Check sheet for the modelled part. Datum: model origin and axes. Units: mm. A direction names the side the tool comes from. Round coordinates to 2 decimals unless told otherwise and drop trailing zeros. Order: outer loops, then holes, each group sorted by start corner. A loop starts at its lowest first (then second) coordinate and runs counter-clockwise, first axis right, second up.
(1) Sectioned sample at C-C, the plane y = 215.5. Enter the section's corners in (x, z).
(2) Thickness scan on probe 1 along X at (y, z) = (1386.5, 16); probe 2 along Z at (x, y) = (-38, 834). Record the ranges inside material, lowest first.
(3) Mould release check, pull along Z, two halves, no side actions. Record for faces 1 (the flat face through (-17.742, 806, 3)), 2 (the flat face through (-37, 806, -15.292)), 3 (the flat face through (-37, 806, 23.208)): released by +Z, released by -Z, zero draft, split by the parting line, or undercut.
(4) Sectioned sample at A-A, the plane x = -49. Enter the section's corners in (y, z).
(5) Sectioned sample at B-B, the plane z = 15. Enter the section's corners in (x, y).
(6) Tool access check on faces 4 (the flat face through (-19.242, 806, 3)), 5 (the flat face through (-57.742, 806, 3)). Record the directions out of +Z, -Z, +X, -X, +Y, -Y that give a thin tool (end or side, any length) a straight path to the whole face; none if there is none.
Autodesk Inventor part; units mm, degrees
ref_plane "YZ Plane" through (0, 0, 0) normal (1, 0, 0) x (0, 1, 0)
ref_plane "XZ Plane" through (0, 0, 0) normal (0, 1, 0) x (-1, 0, 0)
ref_plane "XY Plane" through (0, 0, 0) normal (0, 0, 1) x (1, 0, 0)
sketch "Sketch1" plane through (0, 0, 0) normal (0, 1, 0) x (-1, 0, 0)
  line L0 (18.2419, 23.2079) -> (57.2419, 23.2079)
  line L1 (57.7419, 22.7079) -> (57.7419, -16.2921)
  line L2 (57.2419, -16.7921) -> (18.2419, -16.7921)
  line L3 (17.7419, -16.2921) -> (17.7419, 22.7079)
  line L4 (56.2419, 21.7079) -> (19.2419, 21.7079)
  line L5 (19.2419, 21.7079) -> (19.2419, -15.2921)
  line L6 (19.2419, -15.2921) -> (56.2419, -15.2921)
  line L7 (56.2419, -15.2921) -> (56.2419, 21.7079)
  arc A0 (18.2419, 23.2079) -> (17.7419, 22.7079) centre (18.2419, 22.7079) ccw
  arc A1 (57.7419, 22.7079) -> (57.2419, 23.2079) centre (57.2419, 22.7079) ccw
  arc A2 (57.2419, -16.7921) -> (57.7419, -16.2921) centre (57.2419, -16.2921) ccw
  arc A3 (17.7419, -16.2921) -> (18.2419, -16.7921) centre (18.2419, -16.2921) ccw
  point P0 (0, 0)
  point P1 (17.7419, 23.2079)
  point P2 (57.7419, 23.2079)
  point P3 (57.7419, -16.7921)
  dimension "d0" = 40
  dimension "d1" = 40
  dimension "d2" = 1.5
  dimension "d3" = 0.5
extrude "Extrusion1" add sketch "Sketch1" along normal blind 1635
properties part number "Metalon_Base_2"
Derived:
1. outline: (-57.74, -16.29) arc R0.5 ccw to (-57.24, -16.79) - (-18.24, -16.79) arc R0.5 ccw to (-17.74, -16.29) - (-17.74, 22.71) arc R0.5 ccw to (-18.24, 23.21) - (-57.24, 23.21) arc R0.5 ccw to (-57.74, 22.71) - close; hole (-56.24, -15.29) - (-19.24, -15.29) - (-19.24, 21.71) - (-56.24, 21.71) - close
2. probe 1: x = -57.74 to -56.24, -19.24 to -17.74
2. probe 2: z = -16.79 to -15.29, 21.71 to 23.21
3. face 1: zero draft
3. face 2: undercut
3. face 3: released by +Z
4. outline: (0, -16.79) - (1635, -16.79) - (1635, -15.29) - (0, -15.29) - close; (0, 21.71) - (1635, 21.71) - (1635, 23.21) - (0, 23.21) - close
5. outline: (-57.74, 0) - (-56.24, 0) - (-56.24, 1635) - (-57.74, 1635) - close; (-19.24, 0) - (-17.74, 0) - (-17.74, 1635) - (-19.24, 1635) - close
6. face 4: +Y, -Y
6. face 5: +Z, -Z, -X, +Y, -Y
